Design review of the part built by this model. Coordinates are the model's own, in mm. Give positions to 0.01 mm unless a question says otherwise; leave off trailing zeros. Loops run counter-clockwise (first coordinate to the right, second up) from the corner with the lowest first, then second, coordinate; pieces in that order, holes last. Notation, with made-up numbers: (-28.5, 56.25) - (12.5, 56.25) arc R15 cw to (12.5, 76.25) - close; hole circle Ø2 at (-30, 68). An arc over 180 degrees is marked (long way). Write each question's results on one line, items separated by ' | '.
from build123d import *

# Parameters (mm, degrees)
F3_R = 6.8209108122
F4_R = 1.6096783158


# Not quite as in the source:
# - a fillet or chamfer that OpenCascade refuses, or shapes differently, is made with other operations: its cross-section is extruded or revolved along the edge and cut away or added


with BuildPart() as f1:
    # F0 (on Front) → F1 (revolve)
    with BuildSketch(Plane.XZ):
        Polygon((-8.3269113675, 0), (0, 0), (0, 15.9264262766), (-1.0918058688, 15.9264262766), (-3.2759886235, 14.8343360052), (-5.3236596286, 10.4659702629), (-4.3680798262, 9.3738790601), (-6.006217096, 8.9643457904), align=None)
    revolve(axis=Axis((0, 0, 7.9632131383), (0, 0, -1)))

    # F2: fillet of radius 5 on 1 edges, made by hand

    # F2_s1 → F2_t2 (revolve, cut)
    with BuildSketch(Plane.XZ):
        with BuildLine():
            ThreePointArc((-4.3680798262, 9.3738790601), (-5.8387408469, 8.0723577213), (-6.6947110993, 6.3048406604))
            Line((-6.6947110993, 6.3048406604), (-6.006217096, 8.9643457904))
            Line((-6.006217096, 8.9643457904), (-4.3680798262, 9.3738790601))
        make_face()
    revolve(axis=Axis((0, 0, 8.9643457904), (0, 0, -1)), mode=Mode.SUBTRACT)

    # F3
    f3_edges = [f1.edges().sort_by_distance(p)[0] for p in [
        (3.275989, 0, 14.834336),
    ]]
    fillet(f3_edges, radius=F3_R)

    # F4
    f4_edges = [f1.edges().sort_by_distance(p)[0] for p in [
        (8.326911, 0, 0),
    ]]
    fillet(f4_edges, radius=F4_R)


solid = f1.part
(1) Insertion check: P1, Ø2, axis at x = 1, y = 5.5, coming from the +Z side; P2, Ø6, axis at x = 3, y = 3, coming from the +Z side; P3, Ø1, axis at y = -5, z = 3.5, coming from the +X side. Each pin has a flat end and moves straight along its axis. Give the tip position at first contact, or say it passes through.
Answers below:
P1: z = 12.03 | P2: z = 15.85 | P3: x = 5.93
(2) Wall thickness on line 1 along Z through (x, y) = (1.75, 1.5); line 2 along X through (y, z) = (-3.75, 1.5); line 3 along Z through (x, y) = (2, 2.75): over which ranges is each line inside the solid? List them lowest first. Write a range as from..to.
Answers below:
line 1: 0..15.17 | line 2: -6.9..6.9 | line 3: 0..14.09
(3) Draft analysis for pull direction Z (two halves, no side actions). For faces 1 (the flat face through (0, 0, 0)), 2 (the conical face through (1.47, -6.6, 6.04)), state which applies: pulls with the +Z half, pulls with the -Z half, needs draft (parallel to the pull), parting line crosses it, or undercut.
Answers below:
face 1: pulls with the -Z half | face 2: pulls with the +Z half
(4) Take a section at A-A on z = 11.25. Give the boundary of the cut face in (x, y), plus the area to 3 significant figures.
Answers below:
outline: circle Ø9.91 at (0, 0) | area: 77.2 mm2
